from build123d import *

# Parameters (mm, degrees)
SKETCH1_W                                       = 38.1
SKETCH1_H                                       = 23.876
GEARBOX_MOUNT_DEPTH                             = 48.26
CBORE_FOR_4_SOCKET_HEAD_CAP_SCREW1_D            = 3.2639
CBORE_FOR_4_SOCKET_HEAD_CAP_SCREW1_DEPTH        = 12.7
CBORE_FOR_4_SOCKET_HEAD_CAP_SCREW1_CBORE_D      = 3.96875
CBORE_FOR_4_SOCKET_HEAD_CAP_SCREW1_CBORE_DEPTH  = 4.7625
CBORE_FOR_4_SOCKET_HEAD_CAP_SCREW1_TIP          = 0.980574487
INSERT_INSTALLATION_CHAMFERS_SIZE               = 0.508
SKETCH7_W                                       = 38.1
SKETCH7_H                                       = 23.876
MOTOR_MOUNT_EXTENSION_DEPTH                     = 41.5798
CBORE_FOR_10_SOCKET_HEAD_CAP_SCREW1_D           = 5.1054
CBORE_FOR_10_SOCKET_HEAD_CAP_SCREW1_CBORE_D     = 9.525
CBORE_FOR_10_SOCKET_HEAD_CAP_SCREW1_CBORE_DEPTH = 4.826
MOTOR_MOUNT_PLATE_DEPTH                         = 6.35
SHAFT_CLEARANCE_REACH                           = 111.391
SKETCH9_R                                       = 4.7625
CSK_FOR_M3_FLAT_HEAD_MACHINE_SCREW1_AT_2_COUNT  = 2
CSK_FOR_M3_FLAT_HEAD_MACHINE_SCREW1_AT_2_PITCH  = 19
CSK_FOR_M3_FLAT_HEAD_MACHINE_SCREW1_AT_3_COUNT  = 2
CSK_FOR_M3_FLAT_HEAD_MACHINE_SCREW1_AT_3_PITCH  = 15.700318468
CSK_FOR_M3_FLAT_HEAD_MACHINE_SCREW1_AT_4_COUNT  = 2
CSK_FOR_M3_FLAT_HEAD_MACHINE_SCREW1_AT_4_PITCH  = 15.700318468
CHAMFER2_SIZE                                   = 12.7


with BuildPart() as part:
    # Sketch1 → Gearbox Mount (new body)
    with BuildSketch(Plane.XY):
        Rectangle(SKETCH1_W, SKETCH1_H)
    extrude(amount=GEARBOX_MOUNT_DEPTH)

    # CBORE for #4 Socket Head Cap Screw1
    with Locations(Plane(origin=(0, 11.938, 0), x_dir=(1, 0, 0), z_dir=(0, 1, 0))):
        with Locations((0, -3.81), (-9.525, -22.225), (0, -40.64), (9.525, -22.225)):
            CounterBoreHole(CBORE_FOR_4_SOCKET_HEAD_CAP_SCREW1_D / 2, CBORE_FOR_4_SOCKET_HEAD_CAP_SCREW1_CBORE_D / 2, CBORE_FOR_4_SOCKET_HEAD_CAP_SCREW1_CBORE_DEPTH, depth=CBORE_FOR_4_SOCKET_HEAD_CAP_SCREW1_DEPTH)
            with Locations((0, 0, -(CBORE_FOR_4_SOCKET_HEAD_CAP_SCREW1_DEPTH + CBORE_FOR_4_SOCKET_HEAD_CAP_SCREW1_TIP / 2))):  # 118° drill point
                Cone(0, CBORE_FOR_4_SOCKET_HEAD_CAP_SCREW1_D / 2, CBORE_FOR_4_SOCKET_HEAD_CAP_SCREW1_TIP, mode=Mode.SUBTRACT)

    # Insert Installation Chamfers
    insert_installation_chamfers_edges = [part.edges().sort_by_distance(p)[0] for p in [
        (7.540625, 11.938, 22.225),
        (-1.984375, 11.938, 40.64),
        (-11.509375, 11.938, 22.225),
        (-1.984375, 11.938, 3.81),
    ]]
    chamfer(insert_installation_chamfers_edges, length=INSERT_INSTALLATION_CHAMFERS_SIZE)

    # Sketch7 → Motor Mount Extension (add)
    with BuildSketch(Plane(origin=(0, 0, 0), x_dir=(-1, 0, 0), z_dir=(0, 0, -1))):
        Rectangle(SKETCH7_W, SKETCH7_H)
    extrude(amount=MOTOR_MOUNT_EXTENSION_DEPTH)

    # CBORE for #10 Socket Head Cap Screw1 (through all)
    with Locations(Plane(origin=(0, 11.938, 0), x_dir=(1, 0, 0), z_dir=(0, 1, 0))):
        with Locations((-9.525, -40.64), (9.525, -40.64), (9.525, -3.81), (-9.525, -3.81)):
            CounterBoreHole(CBORE_FOR_10_SOCKET_HEAD_CAP_SCREW1_D / 2, CBORE_FOR_10_SOCKET_HEAD_CAP_SCREW1_CBORE_D / 2, CBORE_FOR_10_SOCKET_HEAD_CAP_SCREW1_CBORE_DEPTH)

    # Sketch8 → Motor Mount Plate (add)
    with BuildSketch(Plane(origin=(0, 0, -41.5798), x_dir=(-1, 0, 0), z_dir=(0, 0, -1))):
        with BuildLine():
            Line((19.05, 11.938), (-19.05, 11.938))
            Line((-19.05, 11.938), (-19.05, -11.938))
            Line((-19.05, -11.938), (-17.446279027, -32.358163541))
            ThreePointArc((-17.446279027, -32.358163541), (0, -48.488), (17.446279027, -32.358163541))
            Line((17.446279027, -32.358163541), (19.05, -11.938))
            Line((19.05, -11.938), (19.05, 11.938))
        make_face()
    extrude(amount=MOTOR_MOUNT_PLATE_DEPTH)

    # Sketch9 → Shaft Clearance (cut, up to next)
    with BuildSketch(Plane(origin=(0, 0, -47.9298), x_dir=(-1, 0, 0), z_dir=(0, 0, -1)), mode=Mode.PRIVATE) as shaft_clearance_sk1:
        with Locations((0, -30.988)):
            Circle(SKETCH9_R)
    shaft_clearance_tool1 = extrude(shaft_clearance_sk1.sketch, amount=-SHAFT_CLEARANCE_REACH, mode=Mode.PRIVATE) & part.part
    add(shaft_clearance_tool1.solids().sort_by_distance((0, -30.988, -47.9298))[0], mode=Mode.SUBTRACT)

    # Sketch10 → CSK for M3 Flat Head Machine Screw1 (revolve, cut)
    with BuildSketch(Plane(origin=(9.5, -30.988, -47.9298), x_dir=(0, 1, 0), z_dir=(1, 0, 0))):
        Polygon((0, 0), (0, 6.35), (1.7, 6.35), (1.7, 5.26), (3.15, 3.81), (3.15, 0), align=None)
    csk_for_m3_flat_head_machine_screw1 = revolve(axis=Axis((9.5, -30.988, -54.2798), (0, 0, 1)), mode=Mode.SUBTRACT)

    # CSK for M3 Flat Head Machine Screw1 at 2: CSK for M3 Flat Head Machine Screw1 ×2
    with Locations(*[(-i * CSK_FOR_M3_FLAT_HEAD_MACHINE_SCREW1_AT_2_PITCH, 0, 0) for i in range(1, CSK_FOR_M3_FLAT_HEAD_MACHINE_SCREW1_AT_2_COUNT)]):
        add(csk_for_m3_flat_head_machine_screw1, mode=Mode.SUBTRACT)

    # CSK for M3 Flat Head Machine Screw1 at 3: CSK for M3 Flat Head Machine Screw1 ×2
    with Locations(*[Vector(-0.6050832675335578, 0.7961621941231026, 0) * (i * CSK_FOR_M3_FLAT_HEAD_MACHINE_SCREW1_AT_3_PITCH) for i in range(1, CSK_FOR_M3_FLAT_HEAD_MACHINE_SCREW1_AT_3_COUNT)]):
        add(csk_for_m3_flat_head_machine_screw1, mode=Mode.SUBTRACT)

    # CSK for M3 Flat Head Machine Screw1 at 4: CSK for M3 Flat Head Machine Screw1 ×2
    with Locations(*[Vector(-0.605083267533558, -0.7961621941231024, 0) * (i * CSK_FOR_M3_FLAT_HEAD_MACHINE_SCREW1_AT_4_PITCH) for i in range(1, CSK_FOR_M3_FLAT_HEAD_MACHINE_SCREW1_AT_4_COUNT)]):
        add(csk_for_m3_flat_head_machine_screw1, mode=Mode.SUBTRACT)

    # Chamfer2
    chamfer2_edges = [part.edges().sort_by_distance(p)[0] for p in [
        (0, 11.938, -47.9298),
    ]]
    chamfer(chamfer2_edges, length=CHAMFER2_SIZE)


solid = part.part
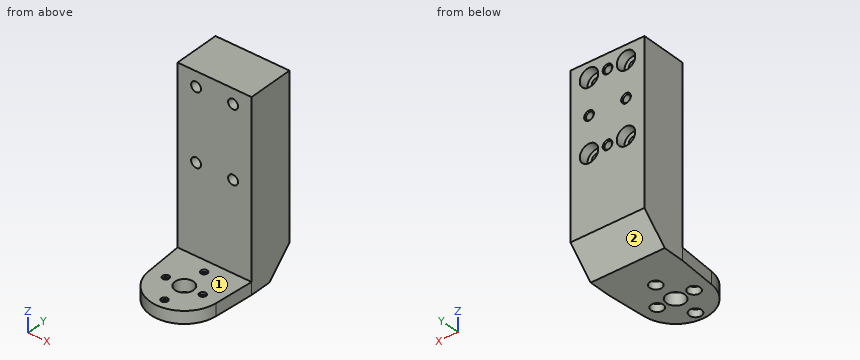
Input: part model. Units: mm. Frame: model coordinates. Face numbers are marked on the shaded views. A direction names the side the tool comes from. Coordinates: 2 decimals unless noted, no trailing zeros. Order: outer loops, then holes, each group sorted by start corner. A loop starts at its lowest first (then second) coordinate and runs counter-clockwise, first axis right, second up. Notation, with made-up numbers: M 33,-26.5 L 72,-26.5 A16 ccw 72,-4.5 Z; hole C 12.25,4.5 d7. An arc over 180 degrees is marked long. Answer in a Markdown table with one row per item.
(1) Section query A-A, the plane y = -3. Output: boundary loops of the cut face in (x, z) (3 decimals), plus the area to 3 significant figures.
Numbers:
| item | result |
|---|---|
| outline | M -19.05,-47.93 L 19.05,-47.93 L 19.05,48.26 L -19.05,48.26 Z; hole C -9.525,3.81 d5.105; hole C -9.525,40.64 d5.105; hole C 9.525,3.81 d5.105; hole C 9.525,40.64 d5.105 |
| area | 3,580 mm^2 |
(2) Material intervals for line 1 (X direction, y = 3, z = 40); line 2 (X direction, y = 8.4, z = 40.64); line 3 (Z direction, x = 8.5, y = -4), sorted ascending. Write a range as [from, to].
Numbers:
| item | result |
|---|---|
| line 1 | x = [-19.05, -12], [-7.05, -1.5], [1.5, 7.05], [12, 19.05] |
| line 2 | x = [-19.05, -14.29], [-4.76, -1.98], [1.98, 4.76], [14.29, 19.05] |
| line 3 | z = [-47.93, 1.47], [6.15, 38.3], [42.98, 48.26] |
(3) Contact query for flat-ended pins moving along their axis: pin 1 Ø3 at (x, z) = (-9.525, 40.64) entering from -Y; pin 2 Ø10 at (x, z) = (13.5, -20.5) entering from -Y; pin 3 Ø5.5 at (x, y) = (-9.5, -30.988) entering from +Z; pin 4 Ø3 at (x, z) = (0.5, 4) entering from +Y. Output: stop coordinate, or through.
Numbers:
| item | result |
|---|---|
| pin 1 | passes through |
| pin 2 | stops at y = -11.94 |
| pin 3 | stops at z = -41.58 |
| pin 4 | stops at y = 11.48 |
(4) Access query for the marked faces 1 and 2. Directions: +Z, -Z, +X, -X, +Y, -Y. A direction counts if a zero-diameter tool reaches every point of the face in a straight line with its end or side. Return the directions, or none.
Numbers:
| item | result |
|---|---|
| face 1 | +Z, +X, -X, -Y |
| face 2 | -Z, +X, -X, +Y |
